from build123d import *

# Parameters (mm, degrees)
ESQUISSE1_W             = 50
ESQUISSE1_H             = 250
BOSS_EXTRU_1_DEPTH      = 5
ESQUISSE2_W             = 5
ESQUISSE2_H             = 250
BOSS_EXTRU_2_DEPTH      = 80
ESQUISSE3_W             = 85
ESQUISSE3_H             = 250
BOSS_EXTRU_3_DEPTH      = 5
ESQUISSE4_W             = 90
ESQUISSE4_H             = 250
BOSS_EXTRU_4_DEPTH      = 5
ESQUISSE5_R             = 10
ENL_V_MAT_EXTRU_1_DEPTH = 5
ESQUISSE6_R             = 5
ENL_V_MAT_EXTRU_2_DEPTH = 5
ESQUISSE8_R             = 20
ESQUISSE8_R_2           = 10
BOSS_EXTRU_5_DEPTH      = 10
ESQUISSE9_W             = 60
ESQUISSE9_H             = 50
ESQUISSE9_R             = 10
BOSS_EXTRU_6_DEPTH      = 10
ESQUISSE11_W            = 90
ESQUISSE11_H            = 10
ENL_V_MAT_EXTRU_6_DEPTH = 271


with BuildPart() as part:
    # Esquisse1 → Boss.-Extru.1 (new body)
    with BuildSketch(Plane.XY):
        with Locations((-25, 125)):
            Rectangle(ESQUISSE1_W, ESQUISSE1_H)
    boss_extru_1 = extrude(amount=BOSS_EXTRU_1_DEPTH)

    # Esquisse2 → Boss.-Extru.2 (add)
    with BuildSketch(Plane.XY.offset(5)):
        with Locations((-47.5, 125)):
            Rectangle(ESQUISSE2_W, ESQUISSE2_H)
    boss_extru_2 = extrude(amount=BOSS_EXTRU_2_DEPTH)

    # Esquisse3 → Boss.-Extru.3 (add)
    with BuildSketch(Plane.XY.offset(85)):
        with Locations((-87.5, 125)):
            Rectangle(ESQUISSE3_W, ESQUISSE3_H)
    boss_extru_3 = extrude(amount=BOSS_EXTRU_3_DEPTH)

    # Esquisse4 → Boss.-Extru.4 (add)
    with BuildSketch(Plane.ZY.offset(130)):
        with Locations((45, 125)):
            Rectangle(ESQUISSE4_W, ESQUISSE4_H)
    boss_extru_4 = extrude(amount=BOSS_EXTRU_4_DEPTH)

    # Esquisse5 → Enlèv. mat.-Extru.1 (cut)
    with BuildSketch(Plane.ZY.offset(50)):
        with Locations((26.5, 125)):
            Circle(ESQUISSE5_R)
    enl_v_mat_extru_1 = extrude(amount=-ENL_V_MAT_EXTRU_1_DEPTH, mode=Mode.SUBTRACT)

    # Esquisse6 → Enlèv. mat.-Extru.2 (cut)
    with BuildSketch(Plane.ZY.offset(50)):
        with Locations((26.5, 205)):
            Circle(ESQUISSE6_R)
        with Locations((26.5, 45)):
            Circle(ESQUISSE6_R)
    enl_v_mat_extru_2 = extrude(amount=-ENL_V_MAT_EXTRU_2_DEPTH, mode=Mode.SUBTRACT)

    # Symétrie2: Boss.-Extru.1, Boss.-Extru.2, Boss.-Extru.3, Boss.-Extru.4, Enlèv. mat.-Extru.1, Enlèv. mat.-Extru.2 across plane
    add(boss_extru_1.mirror(Plane(origin=(0, 0, 5), x_dir=(0, 0, 1), z_dir=(-1, 0, 0))))
    add(boss_extru_2.mirror(Plane(origin=(0, 0, 5), x_dir=(0, 0, 1), z_dir=(-1, 0, 0))))
    add(boss_extru_3.mirror(Plane(origin=(0, 0, 5), x_dir=(0, 0, 1), z_dir=(-1, 0, 0))))
    add(boss_extru_4.mirror(Plane(origin=(0, 0, 5), x_dir=(0, 0, 1), z_dir=(-1, 0, 0))))
    add(enl_v_mat_extru_1.mirror(Plane(origin=(0, 0, 5), x_dir=(0, 0, 1), z_dir=(-1, 0, 0))), mode=Mode.SUBTRACT)
    add(enl_v_mat_extru_2.mirror(Plane(origin=(0, 0, 5), x_dir=(0, 0, 1), z_dir=(-1, 0, 0))), mode=Mode.SUBTRACT)

    # Esquisse8 → Boss.-Extru.5 (add)
    with BuildSketch(Plane(origin=(135, 0, 0), x_dir=(0, 0, -1), z_dir=(1, 0, 0))):
        Polygon((-90, 101.191980235), (-90, 125), (-90, 126.191980235), (-90, 151.191980235), (-150, 151.191980235), (-150, 125), (-150, 101.191980235), align=None)
        with Locations((-110, 126.191980235)):
            Circle(ESQUISSE8_R, mode=Mode.SUBTRACT)
        with Locations((-110, 126.191980235)):
            Circle(ESQUISSE8_R)
        with Locations((-110, 126.191980235)):
            Circle(ESQUISSE8_R_2, mode=Mode.SUBTRACT)
    extrude(amount=-BOSS_EXTRU_5_DEPTH)

    # Esquisse9 → Boss.-Extru.6 (add)
    with BuildSketch(Plane.ZY.offset(135)):
        with Locations((120, 126.191980235)):
            Rectangle(ESQUISSE9_W, ESQUISSE9_H)
        with Locations((110, 126.191980235)):
            Circle(ESQUISSE9_R, mode=Mode.SUBTRACT)
    extrude(amount=-BOSS_EXTRU_6_DEPTH)

    # Esquisse11 → Enlèv. mat.-Extru.6 (cut, through all)
    with BuildSketch(Plane(origin=(135, 0, 0), x_dir=(0, 0, -1), z_dir=(1, 0, 0))):
        with Locations((-45, 5)):
            Rectangle(ESQUISSE11_W, ESQUISSE11_H)
        with Locations((-45, 245)):
            Rectangle(ESQUISSE11_W, ESQUISSE11_H)
    extrude(amount=-ENL_V_MAT_EXTRU_6_DEPTH, mode=Mode.SUBTRACT)


solid = part.part
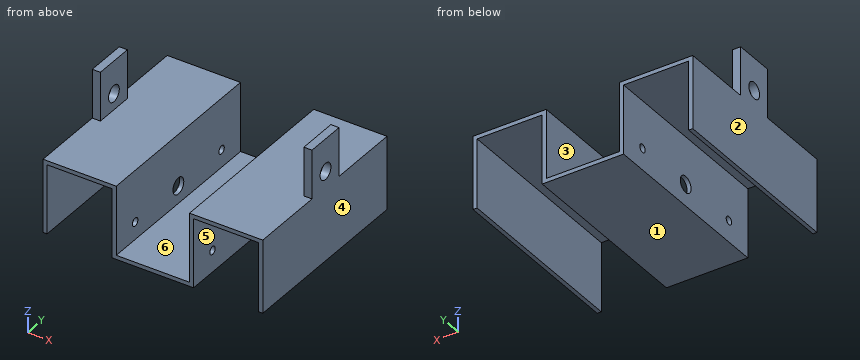
Model file for the job. Use its own axes, mm. Face numbers are marked on the shaded views. A direction names the side the tool comes from. Coordinates: 2 decimals unless noted, no trailing zeros. Write each loop counter-clockwise with the first axis right and the second up, starting at its lowest first coordinate (ties: lowest second). Pieces come first, ordered by that corner, then holes. Notation, with made-up numbers: (59, 79) -> (106, 79) arc R25 cw to (106, 94) -> close; hole circle Ø6 at (33, 79). An arc over 180 degrees is marked (long way). One line per item, written item: value. Start each with the question number.
1) Probe probe 1 along X at (y, z) = (95.5, 51.5); probe 2 along Y at (x, z) = (-48.85, 26.5); probe 3 along Z at (x, y) = (-75, 66). List the from-to ranges inside material, lowest first.
2) Slice it at B-B on z = 110. Write the cut outline in (x, y).
3) Slice it at D-D on y = 28. Write the cut outline in (x, z).
4) Slice it at A-A on y = 205. Write the cut outline in (x, z), then the cut area to 3 significant figures.
5) Slice it at C-C on z = 26.5. Count the separate pieces of the cut face and the enclosed holes in it, then the cut area to 3 significant figures.
6) Pull direction X, two halves, no side cores. Call the marked faces 1, 2 and 3: +X half, -X half, draft (parallel to the pull), parting line (faces both ways), or undercut.
7) Which spindle directions (+Z, -Z, +X, -X, +Y, -Y) get a long thin tool onto all of the face, cutting with end or side? Do the marked faces 4, 5 and 6. Say none if no direction does.
8) Flat gauge pins, fed straight in: pin 1 Ø3 at (x, z) = (129.5, 124) entering from +Y; pin 2 Ø3 at (x, z) = (129.5, 114) entering from -Y; pin 3 Ø10 at (x, y) = (-100.5, 155) entering from +Z. Where does each tip first touch, or does it go through?
Answers follow:
1. probe 1: -135 to -130, -50 to -45, 45 to 50, 130 to 135
1. probe 2: 10 to 40, 50 to 115, 135 to 200, 210 to 240
1. probe 3: 85 to 90
2. outline: (-135, 101.19) -> (-125, 101.19) -> (-125, 116.19) -> (-135, 116.19) -> close; (-135, 136.19) -> (-125, 136.19) -> (-125, 151.19) -> (-135, 151.19) -> close; (125, 101.19) -> (135, 101.19) -> (135, 116.19) -> (125, 116.19) -> close; (125, 136.19) -> (135, 136.19) -> (135, 151.19) -> (125, 151.19) -> close
3. outline: (-135, 0) -> (-130, 0) -> (-130, 85) -> (-50, 85) -> (-50, 0) -> (50, 0) -> (50, 85) -> (130, 85) -> (130, 0) -> (135, 0) -> (135, 90) -> (45, 90) -> (45, 5) -> (-45, 5) -> (-45, 90) -> (-135, 90) -> close
4. outline: (-135, 0) -> (-130, 0) -> (-130, 85) -> (-50, 85) -> (-50, 31.5) -> (-45, 31.5) -> (-45, 90) -> (-135, 90) -> close; (-50, 0) -> (50, 0) -> (50, 21.5) -> (45, 21.5) -> (45, 5) -> (-45, 5) -> (-45, 21.5) -> (-50, 21.5) -> close; (45, 31.5) -> (50, 31.5) -> (50, 85) -> (130, 85) -> (130, 0) -> (135, 0) -> (135, 90) -> (45, 90) -> close
4. area: 2,950 mm2
5. separate pieces: 10
5. enclosed holes: 0
5. area: 4,200 mm2
6. face 1: draft
6. face 2: -X half
6. face 3: undercut
7. face 4: +Z, -Z, +X, +Y, -Y
7. face 5: -Z, +Y, -Y
7. face 6: +Z, +Y, -Y
8. pin 1: y = 151.19
8. pin 2: y = 101.19
8. pin 3: z = 90
